from build123d import *

# Parameters (mm, degrees)
F0_R      = 6
F1_DEPTH  = 5
F2_R      = 6
F3_DEPTH  = 5
F4_R      = 6
F5_DEPTH  = 5
F6_R      = 6
F7_DEPTH  = 5
F8_SIZE2  = 0.2055374144
F8_SIZE   = 2.5
F9_SIZE2  = 1.149871526
F9_SIZE   = 2.5
F10_SIZE2 = 2.8860789389
F10_SIZE  = 2.5
F11_SIZE2 = 0.909916
F11_SIZE  = 2.49999
F12_SIZE2 = 1.809688
F12_SIZE  = 2.49999
F13_SIZE2 = 4.721668
F13_SIZE  = 2.49999


# Not quite as in the source:
# - a fillet or chamfer is up to 0.001 mm smaller than in the source, because OpenCascade refuses the exact size


with BuildPart() as f1:
    # F0 (on Front) → F1 (new body)
    with BuildSketch(Plane.XZ):
        with BuildLine():
            Line((-100, 7.1879485566), (-100, -32.29))
            Line((-100, -32.29), (100, -32.29))
            Line((100, -32.29), (100, 7.1879485566))
            ThreePointArc((100, 7.1879485566), (0, 17.29), (-100, 7.1879485566))
        make_face()
        Circle(F0_R, mode=Mode.SUBTRACT)
    extrude(amount=F1_DEPTH)

    # F2 (on face) → F3 (join)
    with BuildSketch(Plane.XZ.offset(5)):
        with BuildLine():
            Line((-100, -30.49), (100, -30.49))
            Line((100, -30.49), (100, 9.4535179491))
            ThreePointArc((100, 9.4535179491), (0, 19.51), (-100, 9.4535179491))
            Line((-100, 9.4535179491), (-100, -30.49))
        make_face()
        Circle(F2_R, mode=Mode.SUBTRACT)
    extrude(amount=F3_DEPTH)

    # F4 (on face) → F5 (join)
    with BuildSketch(Plane.XZ.offset(10)):
        with BuildLine():
            Line((-100, -26.09), (100, -26.09))
            Line((100, -26.09), (100, 14.2486365081))
            ThreePointArc((100, 14.2486365081), (0, 24.21), (-100, 14.2486365081))
            Line((-100, 14.2486365081), (-100, -26.09))
        make_face()
        Circle(F4_R, mode=Mode.SUBTRACT)
    extrude(amount=F5_DEPTH)

    # F6 (on face) → F7 (join)
    with BuildSketch(Plane.XZ.offset(15)):
        with BuildLine():
            Line((-100, -17.79), (100, -17.79))
            Line((100, -17.79), (100, 22.7020537739))
            ThreePointArc((100, 22.7020537739), (0, 32.5), (-100, 22.7020537739))
            Line((-100, 22.7020537739), (-100, -17.79))
        make_face()
        Circle(F6_R, mode=Mode.SUBTRACT)
    extrude(amount=F7_DEPTH)

    # F8
    f8_edges = [f1.edges().sort_by_distance(p)[0] for p in [
        (0, 0, 17.29),
    ]]
    f8_side = f1.faces().sort_by_distance((0, -2.5, 17.29))[0]
    chamfer(f8_edges, length=F8_SIZE, length2=F8_SIZE2, reference=f8_side)

    # F9
    f9_edges = [f1.edges().sort_by_distance(p)[0] for p in [
        (0, -5, 19.51),
    ]]
    f9_side = f1.faces().sort_by_distance((0, -7.5, 19.51))[0]
    chamfer(f9_edges, length=F9_SIZE, length2=F9_SIZE2, reference=f9_side)

    # F10
    f10_edges = [f1.edges().sort_by_distance(p)[0] for p in [
        (0, -10, 24.21),
    ]]
    f10_side = f1.faces().sort_by_distance((0, -12.5, 24.21))[0]
    chamfer(f10_edges, length=F10_SIZE, length2=F10_SIZE2, reference=f10_side)

    # F11 (size 2.5 and 0.9099255857 in the source; OpenCascade refuses exactly that, so slightly less here)
    f11_edges = [f1.edges().sort_by_distance(p)[0] for p in [
        (0, -5, 17.29),
    ]]
    f11_side = f1.faces().sort_by_distance((0, -3.75, 17.29))[0]
    chamfer(f11_edges, length=F11_SIZE, length2=F11_SIZE2, reference=f11_side)

    # F12 (size 2.5 and 1.8096981916 in the source; OpenCascade refuses exactly that, so slightly less here)
    f12_edges = [f1.edges().sort_by_distance(p)[0] for p in [
        (0, -10, 19.51),
    ]]
    f12_side = f1.faces().sort_by_distance((0, -8.75, 19.51))[0]
    chamfer(f12_edges, length=F12_SIZE, length2=F12_SIZE2, reference=f12_side)

    # F13 (size 2.5 and 4.7216783541 in the source; OpenCascade refuses exactly that, so slightly less here)
    f13_edges = [f1.edges().sort_by_distance(p)[0] for p in [
        (0, -15, 24.21),
    ]]
    f13_side = f1.faces().sort_by_distance((0, -13.75, 24.21))[0]
    chamfer(f13_edges, length=F13_SIZE, length2=F13_SIZE2, reference=f13_side)

    # F14: F1 across plane


with BuildPart() as f1_1:
    add(f1.part)
    add(f1.part.mirror(Plane.XZ))


solid = f1_1.part
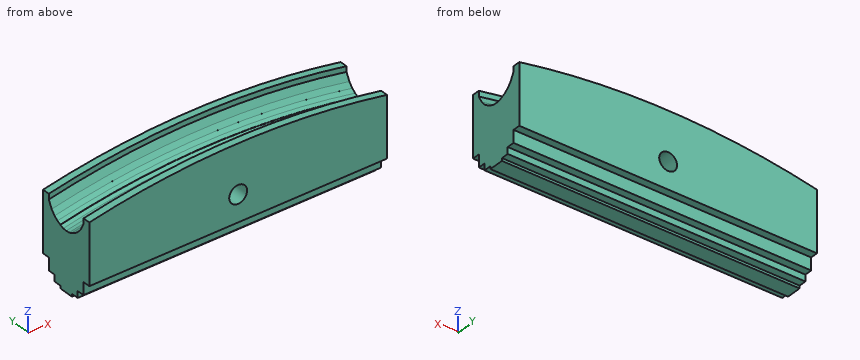
Design review of the part built by this model. Coordinates are the model's own, in mm. Round coordinates to 2 decimals unless told otherwise and drop trailing zeros. Write each loop counter-clockwise with the first axis right and the second up, starting at its lowest first coordinate (ties: lowest second). Pieces come first, ordered by that corner, then holes.
Item 1: Consider section A-A on z = 0. Give the boundary of the cut face in (x, y).
Item 2: Wall thickness on L1, parallel to Y at x = -74.5, z = 23.5; L2, parallel to Z at x = 3.5, y = -12.5; L3, parallel to X at y = -7, z = -3.5: over which ranges is each line inside the solid? List them lowest first.
Item 3: For pin 1 Ø4 at (x, y) = (14, -18.5) entering from -Z; pin 2 Ø4 at (x, z) = (17.5, -21) entering from -Y; pin 3 Ø2.5 at (x, y) = (-8, 8) entering from -Z, all flat-tipped, find the tip position at first contact; note any pin that passes through.
Item 4: Consider section B-B on y = 17. Give the boundary of the cut face in (x, z), and give its area (3 significant figures).
Check values:
1. outline: (-100, -20) - (-6, -20) - (-6, 20) - (-100, 20) - close; (6, -20) - (100, -20) - (100, 20) - (6, 20) - close
2. L1: y = -20 to -15, 15 to 20
2. L2: z = -26.09 to -4.87, 4.87 to 24.2
2. L3: x = -100 to -4.87, 4.87 to 100
3. pin 1: stops at z = -17.79
3. pin 2: stops at y = -15
3. pin 3: stops at z = -30.49
4. outline: (-100, -17.79) - (100, -17.79) - (100, 22.7) arc R515.21 ccw to (-100, 22.7) - close; hole circle Ø12 at (0, 0)
4. area: 9,290 mm2
